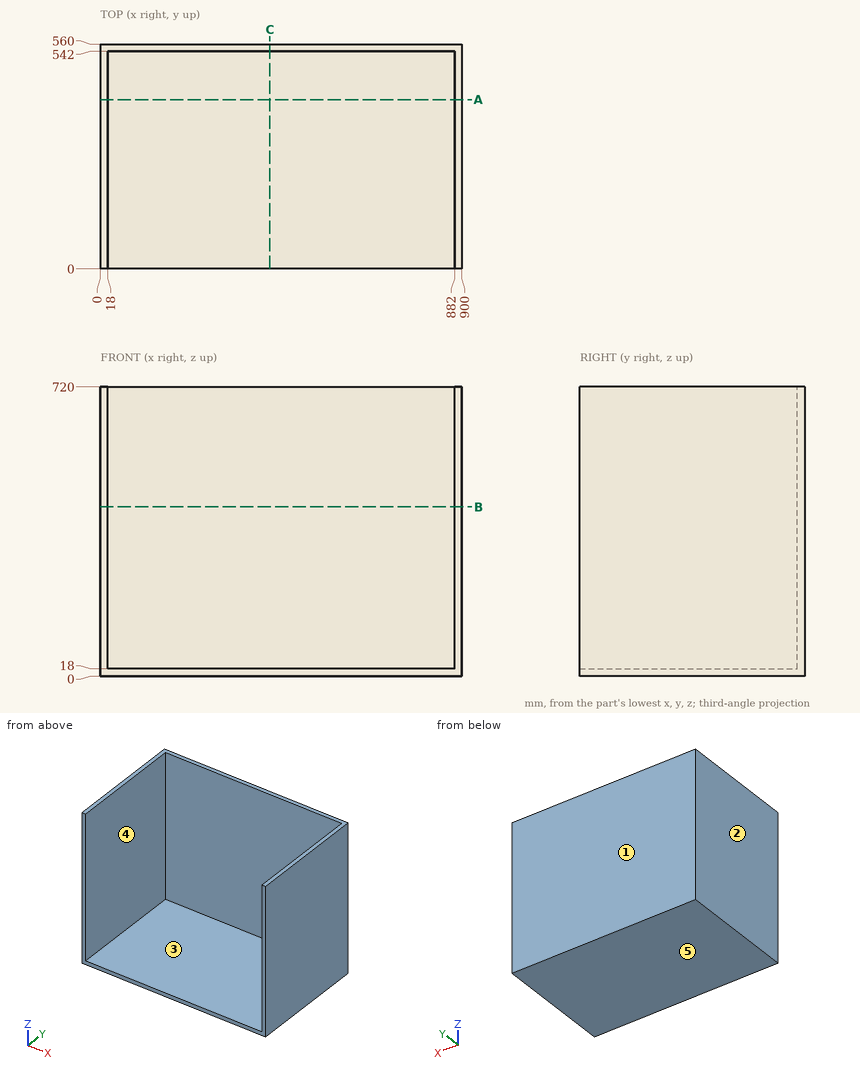
Here's the drawing with two shaded views (mm, measured from the low corner). I have some questions. A direction names the side the tool comes from. Coordinates: 2 decimals unless noted, no trailing zeros. Loops run counter-clockwise (first coordinate to the right, second up) from the corner with the lowest first, then second, coordinate; pieces in that order, holes last. Notation, with made-up numbers: M -30.5,76 L 16.5,76 A31 cw 16.5,108 Z; hole C 85.25,26 d6. An arc over 180 degrees is marked long. Return JSON: item names as keys, results as strings. Group by question number.
Item 1: I'm going to push flat-ended pins straight in: pin 1 Ø5 at (x, y) = (607.5, 340) entering from -Z; pin 2 Ø2 at (x, y) = (324, 285.5) entering from +Z; pin 3 Ø5 at (x, z) = (129, 515) entering from -Y. Where does each tip first touch, or does it pass through?
Item 2: On a 3-axis mill with a long thin cutter (end or side, diameter ignored), from which of +Z, -Z, +X, -X, +Y, -Y can I reach the whole of each face in a straight line? I mean the marked faces 4 and 5. Say none if no direction works.
Item 3: Imagine slicing it at C-C (x = 422). Please give me the cut outline in (y, z), and give its area (3 significant figures).
Item 4: Thinking about a two-plate mould opening in X: for the marked faces 1, 2 and 3, which applies, released by +X, released by -X, zero draft, split by the parting line, or undercut?
Item 5: Imagine slicing it at A-A (y = 421.5). Please give me the cut outline in (x, z), and give its area (3 significant figures).
Item 6: Imagine slicing it at B-B (z = 421). Please give me the cut outline in (x, y), and give its area (3 significant figures).
Item 7: If I drill on L1, parallel to X at y = 212, z = 400.5; L2, parallel to Z at x = 642.5, y = 203; L3, parallel to Y at x = 305, z = 250, over which ranges is the centre line in solid material (lowest first)? Write a range as from..to.
Verdict:
{
 "1": {"pin 1": "stops at z = 0", "pin 2": "stops at z = 18", "pin 3": "stops at y = 542"},
 "2": {"face 4": "+Z, -Y", "face 5": "-Z, +X, -X, +Y, -Y"},
 "3": {"outline": "M 0,0 L 560,0 L 560,720 L 542,720 L 542,18 L 0,18 Z", "area": "22,700 mm^2"},
 "4": {"face 1": "zero draft", "face 2": "released by -X", "face 3": "undercut"},
 "5": {"outline": "M 0,0 L 900,0 L 900,720 L 882,720 L 882,18 L 18,18 L 18,720 L 0,720 Z", "area": "41,500 mm^2"},
 "6": {"outline": "M 0,0 L 18,0 L 18,542 L 882,542 L 882,0 L 900,0 L 900,560 L 0,560 Z", "area": "35,700 mm^2"},
 "7": {"L1": "x = 0..18, 882..900", "L2": "z = 0..18", "L3": "y = 542..560"}
}
